Autodesk Inventor part; units mm, degrees
ref_plane "YZ Plane" through (0, 0, 0) normal (1, 0, 0) x (0, 1, 0)
ref_plane "XZ Plane" through (0, 0, 0) normal (0, 1, 0) x (-1, 0, 0)
ref_plane "XY Plane" through (0, 0, 0) normal (0, 0, 1) x (1, 0, 0)
sketch "スケッチ1" plane through (0, 0, 0) normal (1, 0, 0) x (0, 1, 0)
  line L0 (15, 0) -> (15, -7)
  line L1 (15, -7) -> (18, -7)
  line L2 (26, -32) -> (10, -32)
  line L3 (10, -32) -> (10, 0)
  line L4 (10, 0) -> (15, 0)
  line L5 (0, -38.4) -> (0, 6.4)
  line L6 (18, -7) -> (18, -11)
  line L7 (18, -11) -> (26, -11)
  line L8 (26, -11) -> (26, -32)
  point P0 (0, 0)
  dimension "d0" = 10
  dimension "d1" = 15
  dimension "d2" = 7
  dimension "d3" = 3
  dimension "d10" = 25
  dimension "d11" = 4
  dimension "d12" = 8
revolve "回転1" add sketch "スケッチ1" angle 360 about axis through (0, 0, -10) along (0, 0, 1)
chamfer "面取り1" distance 0.5 angle 45 1 edges at (0, -15, 0)
sketch "スケッチ2" plane through (0, 0, -11) normal (0, 0, 1) x (1, 0, 0)
  circle A0 centre (0, 0) radius 26
  circle A1 centre (0, 0) radius 22
  point P0 (0, 22)
  point P1 (-19.0526, 11)
  point P2 (-19.0526, -11)
  point P3 (0, -22)
  point P4 (19.0526, -11)
  point P5 (19.0526, 11)
  dimension "d13" = 4
  dimension "d16" = 360
hole "穴1" at (0, 22, -11) at (-19.0526, 11, -11) at (-19.0526, -11, -11) at (0, -22, -11) at (19.0526, -11, -11) at (19.0526, 11, -11) direction (0, 0, -1) diameter 3.2 end through all
properties part number "base6" material "ABS プラスチック"
The listing builds one solid part. Answer for the finished solid, in the listing's coordinates (mm). A direction names the side the tool comes from. Coordinates: 2 decimals unless noted, no trailing zeros. Write each loop counter-clockwise with the first axis right and the second up, starting at its lowest first coordinate (ties: lowest second). Pieces come first, ordered by that corner, then holes. Notation, with made-up numbers: (25, 27.5) - (83, 27.5) arc R14 ccw to (83, 48.5) - close; hole circle Ø4 at (80, 47). An arc over 180 degrees is marked (long way). Return JSON: item names as keys, results as strings. Group by question number.
Q1. The part is cut by section C-C on z = -29. Write down the section's boundary in (x, y).
Q2. Flat-ended cylindrical pins translate along their axes: pin 1 Ø5 at (x, z) = (-15, -21) entering from +Y; pin 2 Ø1 at (y, z) = (-20, -28.5) entering from -X; pin 3 Ø5 at (x, y) = (-17.5, -15.5) entering from +Z. Find the tip coordinate at first contact, or state that the pin passes through.
Q3. Find the intervals of material crossed by line 1 along Y through (x, z) = (0, -14); line 2 along X through (y, z) = (-11, -16.5); line 3 along X through (y, z) = (-12, -19), in increasing order. Write a range as [from, to].
Q4. The part is cut by section B-B on z = -6. Write down the section's boundary in (x, y).
Q5. Which of the six approach directions +Z, -Z, +X, -X, +Y, -Y give full straight-line access (tool end or side, diameter ignored) to faces 1 (the flat face through (5, -18, -11)), 2 (the cylindrical face through (-19.1, 12.6, -21.6))?
Q6. For a pull along X with two mould halves and no side action, classify faces 3 (the cylindrical face through (17.847, -2.343, -9.028)), 4 (the cylindrical face through (19, -9.4, -21.6)), 5 (the flat face through (11, 0, -32)) as +X half, -X half, draft (parallel to the pull), parting line (faces both ways), or undercut.
Q7. The part is cut by section D-D on y = 22. Write down the section's boundary in (x, z), and give its area (3 significant figures).
Q8. The part is cut by section A-A on y = 0. Write down the section's boundary in (x, z), and give its area (3 significant figures).
Evaluation:
{
 "1": {"outline": "circle Ø52 at (0, 0); hole circle Ø3.2 at (-19.05, -11); hole circle Ø3.2 at (-19.05, 11); hole circle Ø20 at (0, 0); hole circle Ø3.2 at (0, -22); hole circle Ø3.2 at (0, 22); hole circle Ø3.2 at (19.05, -11); hole circle Ø3.2 at (19.05, 11)"},
 "2": {"pin 1": "stops at y = 22.8", "pin 2": "stops at x = -17.2", "pin 3": "stops at z = -11"},
 "3": {"line 1": "y = [-26, -23.6], [-20.4, -10], [10, 20.4], [23.6, 26]", "line 2": "x = [-23.56, -20.65], [-17.45, 17.45], [20.65, 23.56]", "line 3": "x = [-23.07, -20.3], [-17.8, 17.8], [20.3, 23.07]"},
 "4": {"outline": "circle Ø30 at (0, 0); hole circle Ø20 at (0, 0)"},
 "5": {"face 1": "+Z", "face 2": "+Z, -Z"},
 "6": {"face 3": "parting line", "face 4": "undercut", "face 5": "draft"},
 "7": {"outline": "(-13.86, -32) - (-1.6, -32) - (-1.6, -11) - (-13.86, -11) - close; (1.6, -32) - (13.86, -32) - (13.86, -11) - (1.6, -11) - close", "area": "515 mm2"},
 "8": {"outline": "(-26, -32) - (-10, -32) - (-10, 0) - (-14.5, 0) - (-15, -0.5) - (-15, -7) - (-18, -7) - (-18, -11) - (-26, -11) - close; (10, -32) - (26, -32) - (26, -11) - (18, -11) - (18, -7) - (15, -7) - (15, -0.5) - (14.5, 0) - (10, 0) - close", "area": "806 mm2"}
}
